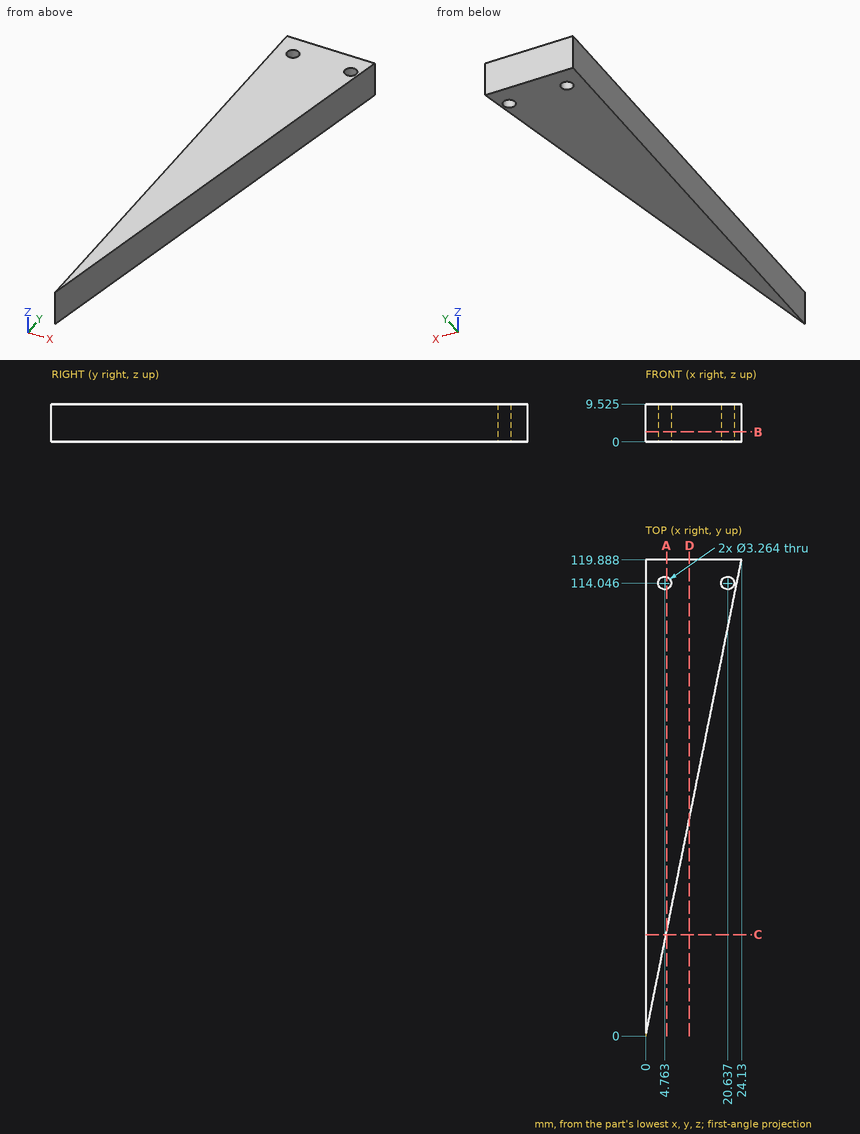
Drawing for the job (mm, zero at the part's lowest x, y, z). Round coordinates to 2 decimals unless told otherwise and drop trailing zeros. Order: outer loops, then holes, each group sorted by start corner. A loop starts at its lowest first (then second) coordinate and runs counter-clockwise, first axis right, second up.
Item 1: Saw through at A-A on x = 5.25. Write the cut outline in (y, z) (1 decimal), then the cut area to 3 significant figures.
Item 2: Pin check, flat tip, straight feed: pin 1 (1 mm diameter, centred on y = 41, z = 4, fed in from +X). Stop position of the tip, or through.
Item 3: Saw through at B-B on z = 2.5. Write the cut outline in (x, y) (1 decimal), then the cut area to 3 significant figures.
Item 4: Saw through at C-C on y = 25.5. Write the cut outline in (x, z) (1 decimal).
Item 5: Probe line 1 along X through (y, z) = (114.5, 9) (1 decimal); line 2 along X through (y, z) = (84.5, 3); line 3 along X through (y, z) = (20.5, 3.5) (1 decimal). List the from-to ranges inside material, lowest first.
Item 6: Saw through at D-D on x = 11. Write the cut outline in (y, z) (1 decimal).
Reported:
1. outline: (26.1, 0) - (112.5, 0) - (112.5, 9.5) - (26.1, 9.5) - close; (115.6, 0) - (119.9, 0) - (119.9, 9.5) - (115.6, 9.5) - close
1. area: 864 mm2
2. pin 1: stops at x = 8.35
3. outline: (0, 0) - (24.1, 119.9) - (0, 119.9) - close; hole circle Ø3.3 at (4.8, 114); hole circle Ø3.3 at (20.6, 114)
3. area: 1,430 mm2
4. outline: (0, 0) - (5.1, 0) - (5.1, 9.5) - (0, 9.5) - close
5. line 1: x = 0 to 3.2, 6.3 to 19.1, 22.2 to 23
5. line 2: x = 0 to 17.01
5. line 3: x = 0 to 4.1
6. outline: (54.7, 0) - (119.9, 0) - (119.9, 9.5) - (54.7, 9.5) - close
